Part model, mm, in its own coordinate system. Coordinates: 2 decimals unless noted, no trailing zeros. Write each loop counter-clockwise with the first axis right and the second up, starting at its lowest first coordinate (ties: lowest second). Pieces come first, ordered by that corner, then holes. Notation, with made-up numbers: M -1,57 L 33,57 A20 ccw 33,89 Z; hole C 9.25,30 d4. An arc over 180 degrees is marked long. Use a Markdown table: item, result. Add a question column.
Q1. Slice it at C-C on x = 0.25. Write the cut outline in (y, z).
Q2. Mould opens along Y. For faces 1 (the flat face through (4, 5, 2)), 2 (the cylindrical face through (-0.221, 9.686, 1.972)), 3 (the flat face through (0, 12, 2)) say: released by +Y, released by -Y, zero draft, split by the parting line, or undercut.
Q3. Pin check, flat tip, straight feed: pin 1 Ø2 at (x, y) = (0, 8) entering from -Z. Stop position of the tip, or through.
Q4. Wall check: L1, parallel to Y at x = 0, z = 0.9 (3 decimals); L2, parallel to Y at x = 0.75, z = 0.7; L3, parallel to X at y = 0, z = 1.35 (3 decimals). Give the ranges that are in metal, low to high. Write a range as from..to.
Q5. Slice it at D-D on x = -2. Write the cut outline in (y, z).
Q6. Slice it at B-B on z = 1.3. Write the cut outline in (x, y) (3 decimals).
Q7. Slice it at A-A on y = 8. Write the cut outline in (x, z).
from build123d import *

# Parameters (mm, degrees)
SKETCH1_R           = 4
BOSS_EXTRUDE1_DEPTH = 4
SKETCH3_W           = 8
SKETCH3_H           = 12
BOSS_EXTRUDE2_DEPTH = 4
SKETCH2_R           = 2.325
CUT_EXTRUDE2_DEPTH  = 5
SKETCH4_R           = 1.7
CUT_EXTRUDE3_DEPTH  = 4
FILLET1_R           = 2.5


with BuildPart() as part:
    # Sketch1 → Boss-Extrude1 (new body)
    with BuildSketch(Plane.XY):
        Circle(SKETCH1_R)
    extrude(amount=BOSS_EXTRUDE1_DEPTH)

    # Sketch3 → Boss-Extrude2 (add)
    with BuildSketch(Plane.XY):
        with Locations((0, 6)):
            Rectangle(SKETCH3_W, SKETCH3_H)
    extrude(amount=BOSS_EXTRUDE2_DEPTH)

    # Sketch2 → Cut-Extrude2 (cut, through all)
    with BuildSketch(Plane.XY):
        Circle(SKETCH2_R)
    extrude(amount=CUT_EXTRUDE2_DEPTH, mode=Mode.SUBTRACT)

    # Sketch4 → Cut-Extrude3 (cut)
    with BuildSketch(Plane.XY):
        with Locations((0, 8)):
            Circle(SKETCH4_R)
    extrude(amount=CUT_EXTRUDE3_DEPTH, mode=Mode.SUBTRACT)

    # Fillet1
    fillet1_edges = [part.edges().sort_by_distance(p)[0] for p in [
        (4, 12, 2),
        (-4, 12, 2),
    ]]
    fillet(fillet1_edges, radius=FILLET1_R)


solid = part.part
Recorded:
| question | item | result |
|---|---|---|
| 1 | outline | M -3.99,0 L -2.31,0 L -2.31,4 L -3.99,4 Z; M 2.31,0 L 6.32,0 L 6.32,4 L 2.31,4 Z; M 9.68,0 L 12,0 L 12,4 L 9.68,4 Z |
| 2 | face 1 | zero draft |
| 2 | face 2 | undercut |
| 2 | face 3 | released by +Y |
| 3 | pin 1 | through |
| 4 | L1 | -4..-2.325, 2.325..6.3, 9.7..12 |
| 4 | L2 | -3.93..-2.2, 2.2..6.47, 9.53..12 |
| 4 | L3 | -4..-2.325, 2.325..4 |
| 5 | outline | M -3.46,0 L -1.19,0 L -1.19,4 L -3.46,4 Z; M 1.19,0 L 11.95,0 L 11.95,4 L 1.19,4 Z |
| 6 | outline | M -4,0 A4 ccw 4,0 L 4,9.5 A2.5 ccw 1.5,12 L -1.5,12 A2.5 ccw -4,9.5 Z; hole C 0,0 d4.65; hole C 0,8 d3.4 |
| 7 | outline | M -4,0 L -1.7,0 L -1.7,4 L -4,4 Z; M 1.7,0 L 4,0 L 4,4 L 1.7,4 Z |
